Check sheet for the drawn part. Datum: minimum x, y, z corner. Units: mm. Round coordinates to 2 decimals unless told otherwise and drop trailing zeros. Write each loop counter-clockwise with the first axis right and the second up, starting at its lowest first coordinate (ties: lowest second). Pieces come first, ordered by that corner, then holes. Notation, with made-up numbers: (-21.75, 54.25) - (11.25, 54.25) arc R27 cw to (11.25, 81.25) - close; hole circle Ø8 at (-35.75, 33). An arc over 180 degrees is marked (long way). Answer as a JSON object with one key per item and string values.
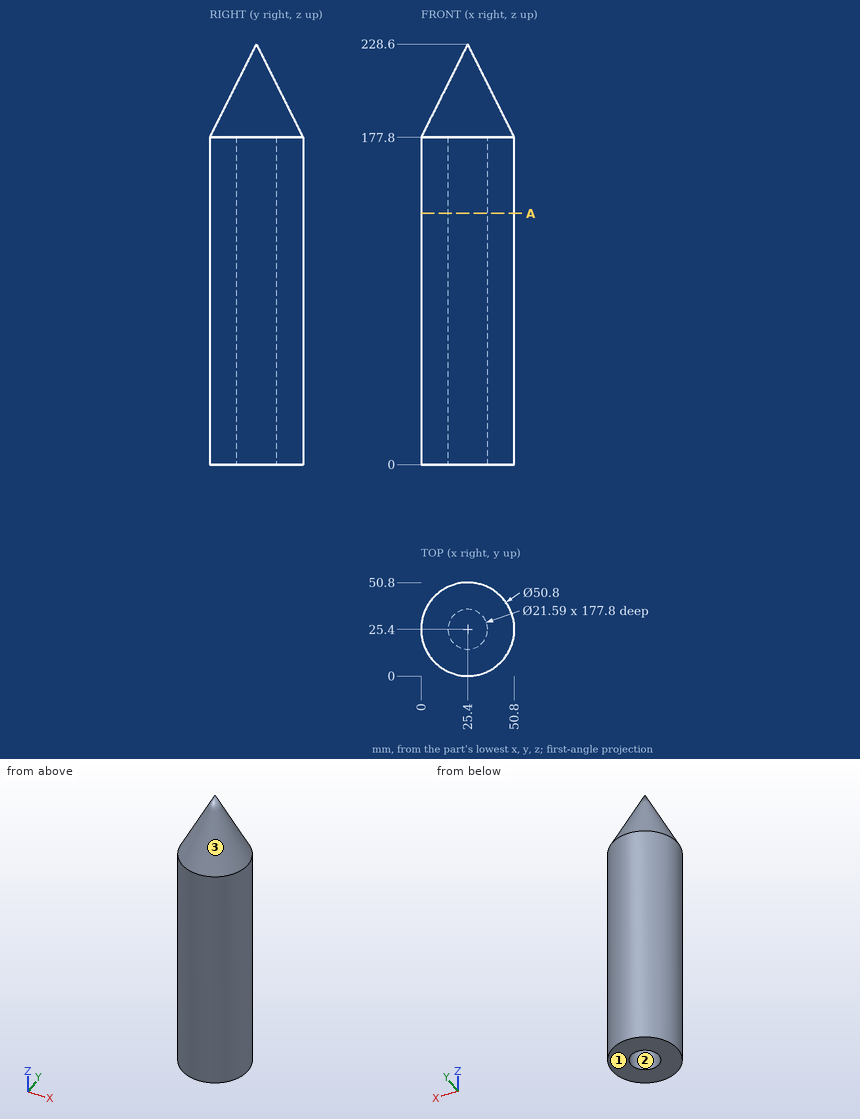
1. Cross-section at A-A (z = 136.5). Record the boundary of the cut face in (x, y) (3 decimals).
Completed:
{"outline": "circle Ø50.8 at (25.4, 25.4); hole circle Ø21.59 at (25.4, 25.4)"}
2. Mould release check, pull along X, two halves, no side actions. Record for the marked faces 1, 2 and 3: released by +X, released by -X, zero draft, split by the parting line, or undercut.
Completed:
{"face 1": "zero draft", "face 2": "undercut", "face 3": "split by the parting line"}
3. Go/stop test with flat-tipped pins: pin 1 (1.5 mm diameter, centred on y = 34.5, z = 188, fed in from +X); pin 2 (1 mm diameter, centred on x = 19, y = 28.5, fed in from -Z); pin 3 (5 mm diameter, centred on x = 17, z = 193, fed in from -Y). Record where each tip stops, or that it passes through.
Completed:
{"pin 1": "stops at x = 44.1", "pin 2": "stops at z = 177.8", "pin 3": "stops at y = 7.91"}
4. Material ranges on probe 1 along Y at (x, z) = (25, 92); probe 2 along X at (y, z) = (31, 110), recorded low to high. Write a range as from..to.
Completed:
{"probe 1": "y = 0..14.61, 36.19..50.8", "probe 2": "x = 0.63..16.17, 34.63..50.17"}
